Here's how the part is built. I have some questions about the finished solid (model axes, mm). A direction names the side the tool comes from. Coordinates: 2 decimals unless noted, no trailing zeros. Write each loop counter-clockwise with the first axis right and the second up, starting at its lowest first coordinate (ties: lowest second). Pieces come first, ordered by that corner, then holes.
Item 1: If we section it at A-A (y = 0): Please give me the cut outline in (x, z).
Item 2: I'm going to push a flat-ended pin straight in: pin 1 Ø18 at (x, y) = (-9.5, -7) entering from +Z. Where does the tip first touch, or does it pass through?
Item 3: If we section it at B-B (x = 57.5): Please give me the cut outline in (y, z).
Item 4: If I drill on line 1 (Y direction, x = -57.5, z = 1.6); line 2 (Y direction, x = -38, z = 2); line 3 (Z direction, x = -54, y = -2.5), over which ranges is the centre line in solid material (lowest first)?
Item 5: For faces 1 (the face through (-50.25, -25, 14)), 2 (the face through (58, 25, 24.2)), 3 (the face through (58, 20, 14)), which set-ups out of +Z, -Z, +X, -X, +Y, -Y let a thin tool reach every point of the face, with its end or its side?
Item 6: We'd pull the mould along X, two halves only. Please class faces 4 (the face through (-50.25, 25, 14)), 5 (the face through (-65, -7, 4)), 6 (the face through (50.25, -25, 14)), 7 (the face through (-1, 0, 0)): +X half, -X half, draft (parallel to the pull), parting line (faces both ways), or undercut.
Item 7: If we section it at C-C (z = 8.25): Please give me the cut outline in (x, y), then the cut area to 3 significant figures.
Item 8: If we section it at D-D (x = -35): Please give me the cut outline in (y, z).
from build123d import *

# Parameters (mm, degrees)
F0_W           = 130
F0_H           = 60
F1_DEPTH       = 4.2
F2_W           = 14.75
F2_H           = 10
F3_DEPTH       = 20
F5_D           = 6.8
F7_D           = 6
F7_CSINK_D     = 15
F7_CSINK_ANGLE = 90
F8_SIZE        = 1


with BuildPart() as f1:
    # F0 (on Top) → F1 (new body)
    with BuildSketch(Plane.XY):
        Rectangle(F0_W, F0_H)
    extrude(amount=F1_DEPTH)

    # F2 (on face) → F3 (join)
    with BuildSketch(Plane.XY.offset(4.2)):
        with Locations((-57.625, 25)):
            Rectangle(F2_W, F2_H)
        with Locations((-57.625, -25)):
            Rectangle(F2_W, F2_H)
        with Locations((57.625, -25)):
            Rectangle(F2_W, F2_H)
        with Locations((57.625, 25)):
            Rectangle(F2_W, F2_H)
    extrude(amount=F3_DEPTH)

    # F5 (through all)
    with Locations(Plane.XY.offset(4.2)):
        with Locations((57.5, 0), (-57.5, 0)):
            Hole(F5_D / 2)

    # F7 (through all)
    with Locations(Plane.XY.offset(4.2)):
        with Locations((35, 0), (-35, 0)):
            CounterSinkHole(F7_D / 2, F7_CSINK_D / 2, counter_sink_angle=F7_CSINK_ANGLE)

    # F8
    f8_edges = [f1.edges().sort_by_distance(p)[0] for p in [
        (-50.25, -25, 24.2),
        (-57.625, -30, 24.2),
        (-65, -25, 24.2),
        (-57.625, -20, 24.2),
        (-57.625, 30, 24.2),
        (-65, 25, 24.2),
        (-57.625, 20, 24.2),
        (-50.25, 25, 24.2),
        (65, -25, 24.2),
        (57.625, -20, 24.2),
        (50.25, -25, 24.2),
        (57.625, -30, 24.2),
        (57.625, 30, 24.2),
        (50.25, 25, 24.2),
        (57.625, 20, 24.2),
        (65, 25, 24.2),
    ]]
    chamfer(f8_edges, length=F8_SIZE)


solid = f1.part
Answer list:
1. outline: (-65, 0) - (-60.9, 0) - (-60.9, 4.2) - (-65, 4.2) - close; (-54.1, 0) - (-38.3, 0) - (-42.5, 4.2) - (-54.1, 4.2) - close; (-31.7, 0) - (31.7, 0) - (27.5, 4.2) - (-27.5, 4.2) - close; (38.3, 0) - (54.1, 0) - (54.1, 4.2) - (42.5, 4.2) - close; (60.9, 0) - (65, 0) - (65, 4.2) - (60.9, 4.2) - close
2. pin 1: stops at z = 4.2
3. outline: (-30, 0) - (-3.4, 0) - (-3.4, 4.2) - (-20, 4.2) - (-20, 23.2) - (-21, 24.2) - (-29, 24.2) - (-30, 23.2) - close; (3.4, 0) - (30, 0) - (30, 23.2) - (29, 24.2) - (21, 24.2) - (20, 23.2) - (20, 4.2) - (3.4, 4.2) - close
4. line 1: y = -30 to -3.4, 3.4 to 30
4. line 2: y = -30 to -4.37, 4.37 to 30
4. line 3: z = 0 to 4.2
5. face 1: +Z, +Y, -Y
5. face 2: +Z, +X, -X, +Y, -Y
5. face 3: +Z, +X, -X
6. face 4: undercut
6. face 5: -X half
6. face 6: undercut
6. face 7: draft
7. outline: (-65, -30) - (-50.25, -30) - (-50.25, -20) - (-65, -20) - close; (-65, 20) - (-50.25, 20) - (-50.25, 30) - (-65, 30) - close; (50.25, -30) - (65, -30) - (65, -20) - (50.25, -20) - close; (50.25, 20) - (65, 20) - (65, 30) - (50.25, 30) - close
7. area: 590 mm2
8. outline: (-30, 0) - (-3.3, 0) - (-7.5, 4.2) - (-30, 4.2) - close; (3.3, 0) - (30, 0) - (30, 4.2) - (7.5, 4.2) - close
